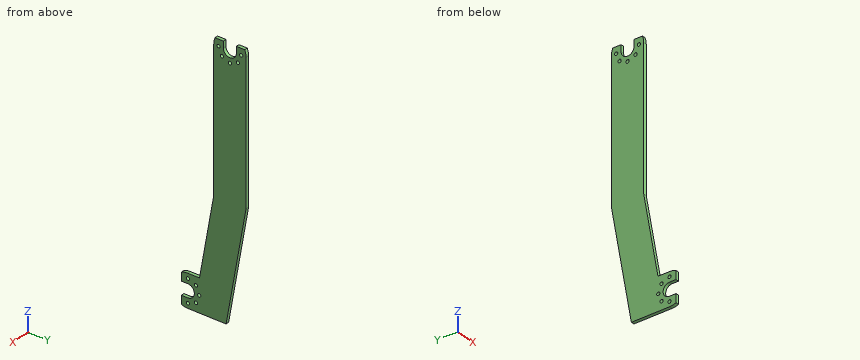
Autodesk Inventor part; units mm, degrees
ref_plane "YZ Plane" through (0, 0, 0) normal (1, 0, 0) x (0, 1, 0)
ref_plane "XZ Plane" through (0, 0, 0) normal (0, 1, 0) x (-1, 0, 0)
ref_plane "XY Plane" through (0, 0, 0) normal (0, 0, 1) x (1, 0, 0)
sketch "スケッチ1" plane through (0, 0, 0) normal (1, 0, 0) x (0, 1, 0)
  line L0 (-20, 80) -> (20, 80)
  line L1 (20, 80) -> (20, -80)
  line L2 (20, -80) -> (-20, -80)
  line L3 (-20, -80) -> (-20, 80)
  point P0 (0, 0)
  dimension "d0" = 160
  dimension "d2" = 40
  dimension "d3" = 20
  dimension "d4" = 80
extrude "押し出し1" add sketch "スケッチ1" along normal blind 2
sketch "スケッチ3" plane through (0, 0, 0) normal (-1, 0, 0) x (0, 0, 1)
  line L0 (80, -20) -> (80, 20)
  line L1 (80, 20) -> (-80, 20)
  line L2 (-80, 20) -> (-80, -20)
  line L3 (-80, -20) -> (80, -20)
  line L4 (-60, -20) -> (-60, -8.8163)
  line L5 (-60, -8.8163) -> (-10, 0)
  line L6 (-10, 0) -> (80, 0)
  line L7 (80, 0) -> (80, 20)
  line L8 (-80, 7.6571) -> (-10, 20)
  point P0 (0, 0)
  dimension "d11" = 20
  dimension "d12" = 10
  dimension "d13" = 10
  dimension "d14" = 20
  dimension "d15" = 160
  dimension "d17" = 90
  dimension "d18" = 90
extrude "押し出し3" cut sketch "スケッチ3" against normal blind 20 contours L6 L5 L4 L3 L2 L8 L1 L0 keep common part
sketch "スケッチ6" plane through (0, 0, 0) normal (-1, 0, 0) x (0, 0, 1)
  line L0 (-60, -8.8163) -> (-60, -20)
  line L1 (-10, 0) -> (-60, -8.8163)
  line L2 (80, 0) -> (-10, 0)
  line L3 (80, 0) -> (80, 20)
  line L4 (80, 20) -> (-10, 20)
  line L5 (-80, 7.6571) -> (-10, 20)
  line L6 (-80, 7.6571) -> (-80, -20)
  line L7 (-80, -20) -> (-60, -20)
  arc A0 (-66, -16) -> (-74, -16) centre (-70, -16) ccw
  arc A1 (76, 14) -> (76, 6) centre (76, 10) ccw
  line L8 (-74, -16) -> (-74, -20)
  line L9 (-66, -16) -> (-66, -20)
  line L10 (76, 14) -> (80, 14)
  line L11 (76, 6) -> (80, 6)
  arc A2 (-60.8348, -20) -> (-60, -16) centre (-70, -16) ccw
  arc A3 (-80, -16) -> (-79.1652, -20) centre (-70, -16) ccw
  arc A4 (76, 0) -> (80, 0.8348) centre (76, 10) ccw
  arc A5 (80, 19.1652) -> (76, 20) centre (76, 10) ccw
  point P0 (0, 0)
  dimension "d39" = 8
  dimension "d40" = 4
  dimension "d41" = 4
  dimension "d42" = 10
  dimension "d43" = 10
extrude "押し出し6" cut sketch "スケッチ6" against normal blind 11 contours L0 A2 L7 L9 A0 L8 A3 L6 L5 L4 A5 L3 L10 A1 L11 A4 L2 L1 keep common part
sketch "スケッチ7" plane through (0, 0, 0) normal (-1, 0, 0) x (0, 0, 1)
  arc A0 (80, 19.1652) -> (76, 20) centre (76, 10) ccw
  arc A1 (-80, -16) -> (-79.1652, -20) centre (-70, -16) ccw
  line L0 (-79.1652, -20) -> (-74, -20)
  line L1 (80, 0.8348) -> (80, 6)
  circle A2 centre (76, 3) radius 1
  circle A3 centre (-77, -16) radius 1
  point P0 (0, 0)
  dimension "d46" = 2
  dimension "d48" = 7
  dimension "d49" = 4
  dimension "d50" = 4
  dimension "d51" = 7
hole "穴1" at (0, -16, -77) at (0, 3, 76) direction (1, 0, 0) diameter 2 end through all
pattern_circular "円形状パターン1" count 5 over 180 about axis through (0, -16, -70) along (1, 0, 0) of "穴1"
pattern_circular "円形状パターン2" count 5 over 180 about axis through (0, 10, 76) along (1, 0, 0) of "穴1"
properties part number "10" material "アルミニウム 6061"
Here's how the part is built. I have some questions about the finished solid (model axes, mm). Coordinates: 2 decimals unless noted, no trailing zeros. Write each loop counter-clockwise with the first axis right and the second up, starting at its lowest first coordinate (ties: lowest second). Pieces come first, ordered by that corner, then holes. Notation, with made-up numbers: M 59,58.25 L 70,58.25 A27 cw 70,74.25 Z; hole C 54,-16.5 d11. An arc over 180 degrees is marked long. Answer as CSV lines item,"result". Start each with the question number.
Q1. Will these pins go through, and if not, where does the flat tip stop? pin 1 Ø1.6 at (y, z) = (-9, -70) entering from -X; pin 2 Ø1 at (x, z) = (0.5, 78) entering from +Y; pin 3 Ø1 at (x, y) = (1, -17.5) entering from +Z.
Q2. Suppose I cut it at B-B, the plane z = -3. List the corners of the cut face in (x, y) for me.
Q3. I need wall thicknesses on probe 1 along Y at (x, z) = (1.4, 76); probe 2 along Z at (x, y) = (0.75, -10.5); probe 3 along Y at (x, z) = (1.05, 14). Which ranges of each line are inside material? Lowest first, please. Write a range as [from, to].
Entries:
1,pin 1,"passes through"
1,pin 2,"stops at y = 19.89"
1,pin 3,"stops at z = -60.05"
2,outline,"M 0,0 L 2,0 L 2,20 L 0,20 Z"
3,probe 1,"y = [0, 2], [4, 6], [14, 16], [18, 20]"
3,probe 2,"z = [-80, -75.78], [-74.11, -65.89], [-64.22, -60]"
3,probe 3,"y = [0, 20]"
